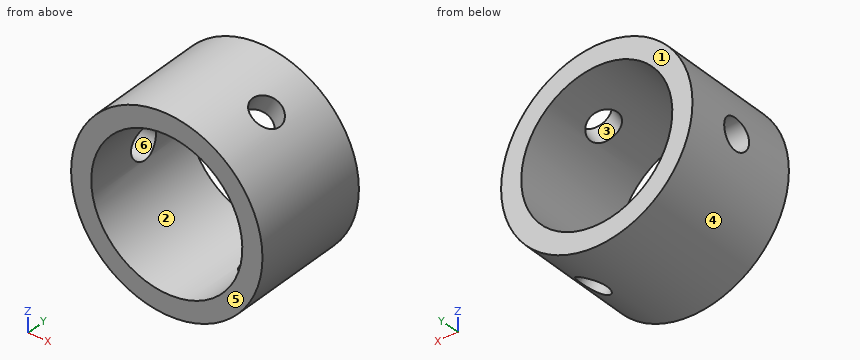
```python
from build123d import *

# Parameters (mm, degrees)
SKETCH_1_R               = 9.5
SKETCH_1_R_2             = 7.5
EXTRUDE_1_DEPTH          = 12
CUT_EXTRUDE_1_REACH      = 20.014
CUT_EXTRUDE_1_END_RADIUS = 9.5
SKETCH_2_R               = 1.55
PATTERN_CIRCULAR_1_COUNT = 3


with BuildPart() as part:
    # 草图1 → 凸台-拉伸1 (new body)
    with BuildSketch(Plane(origin=(0, 0, 0), x_dir=(1, 0, 0), z_dir=(0, 1, 0))):
        with Locations(Location((0, 0, 0), (0, 0, 270))):
            Circle(SKETCH_1_R)
        with Locations(Location((0, 0, 0), (0, 0, 270))):
            Circle(SKETCH_1_R_2, mode=Mode.SUBTRACT)
    extrude(amount=EXTRUDE_1_DEPTH)

    # 切除-拉伸1: up to this cylinder (the profile starts inside it)
    cut_extrude_1_end = Plane(origin=(0, 6.5, 0), z_dir=(0, -1, 0)) * Cylinder(CUT_EXTRUDE_1_END_RADIUS, 60.028, mode=Mode.PRIVATE)
    # 草图2 → 切除-拉伸1 (cut, up to the surface)
    with BuildSketch(Plane(origin=(0, 0, 0), x_dir=(0, 0, -1), z_dir=(1, 0, 0)), mode=Mode.PRIVATE) as cut_extrude_1_sk1:
        with Locations((0, 6.5)):
            Circle(SKETCH_2_R)
    cut_extrude_1_tool1 = extrude(cut_extrude_1_sk1.sketch, amount=-CUT_EXTRUDE_1_REACH, mode=Mode.PRIVATE) & cut_extrude_1_end
    cut_extrude_1 = cut_extrude_1_tool1.solids().sort_by_distance((0, 6.5, 0))[0]
    add(cut_extrude_1, mode=Mode.SUBTRACT)

    # 阵列(圆周)1: 切除-拉伸1 ×3 about axis
    pattern_circular_1_axis = Axis((0, 12, 0), (0, 1, 0))
    for i in range(1, PATTERN_CIRCULAR_1_COUNT):
        add(cut_extrude_1.rotate(pattern_circular_1_axis, i * 360 / PATTERN_CIRCULAR_1_COUNT), mode=Mode.SUBTRACT)


solid = part.part
```
Input: part model. Units: mm. Frame: model coordinates. Face numbers are marked on the shaded views. A direction names the side the tool comes from. Round coordinates to 2 decimals unless told otherwise and drop trailing zeros. Write each loop counter-clockwise with the first axis right and the second up, starting at its lowest first coordinate (ties: lowest second). Pieces come first, ordered by that corner, then holes. Notation, with made-up numbers: M -6.5,86.25 L 25.5,86.25 A22 ccw 25.5,108.25 Z; hole C -33,16.5 d9. An arc over 180 degrees is marked long. Write each question's results on one line, items separated by ' | '.
Q1. Access query for the marked faces 5 and 6. Directions: +Z, -Z, +X, -X, +Y, -Y. A direction counts if a zero-diameter tool reaches every point of the face in a straight line with its end or side. Return the directions, or none.
Results:
face 5: +Z, -Z, +X, -X, -Y | face 6: -X
Q2. Section query C-C (y = 7). Return loops of the section in (x, z).
Results:
outline: M -9.39,-1.47 A9.5 ccw 3.42,-8.86 L 2.41,-7.1 A7.5 cw -7.36,-1.47 Z; M -9.39,1.47 L -7.36,1.47 A7.5 cw 2.41,7.1 L 3.42,8.86 A9.5 ccw Z; M 4.95,-5.64 L 5.96,-7.39 A9.5 ccw 5.96,7.39 L 4.95,5.64 A7.5 cw Z
Q3. Section query B-B (z = 0). Return loops of the section in (x, y), and give its area (3 significant figures).
Results:
outline: M -9.5,0 L -7.5,0 L -7.5,4.95 L -9.5,4.95 Z; M -9.5,8.05 L -7.5,8.05 L -7.5,12 L -9.5,12 Z; M 7.5,0 L 9.5,0 L 9.5,12 L 7.5,12 Z | area: 41.8 mm^2
Q4. Section query A-A (x = 0). Return loops of the section in (y, z).
Results:
outline: M 0,-9.5 L 12,-9.5 L 12,-7.5 L 0,-7.5 Z; M 0,7.5 L 12,7.5 L 12,9.5 L 0,9.5 Z
Q5. Line query: line 1 along Y through (x, z) = (-8.5, 0); line 2 along X through (y, z) = (9, 0); line 3 along Y through (x, z) = (4, 8.5). Output: solid intervals per line, ascending.
Results:
line 1: y = 0 to 4.95, 8.05 to 12 | line 2: x = -9.5 to -7.5, 7.5 to 9.5 | line 3: y = 0 to 5.16, 7.84 to 12
Q6. Section query D-D (z = 4.75). Return loops of the section in (x, y).
Results:
outline: M -8.23,0 L -5.8,0 L -5.8,12 L -8.23,12 Z; M 5.8,0 L 8.23,0 L 8.23,12 L 5.8,12 Z
Q7. Draft query along X for the marked faces 1, 2, 3 and 4. Return one class per face: released by +X, released by -X, zero draft, split by the parting line, or undercut.
Results:
face 1: zero draft | face 2: undercut | face 3: undercut | face 4: split by the parting line
Q8. Pin query (flat end, axial travel): P1, Ø1, axis at x = 2.5, y = 2.5, coming from the -Z side. Return the tip coordinate at first contact, or that it passes through.
Results:
P1: stops at z = -9.29
